Autodesk Inventor part; units mm, degrees
ref_plane "FDT_MOUNT_XY" through (0, 0, 8) normal (0, 0, 1) x (0, 1, 0)
ref_plane "FDT_MOUNT_YZ" through (0, 0, 8) normal (0, 1, 0) x (-1, 0, 0)
ref_plane "FDT_MOUNT_ZX" through (0, 0, 8) normal (-1, 0, 0) x (0, 0, 1)
sketch "Skizze_1" plane through (0, 0, 0) normal (0, 0, 1) x (1, 0, 0)
  line L0 (-14, 25) -> (-14, -25)
  line L1 (-14, -25) -> (14, -25)
  line L2 (14, -25) -> (14, 25)
  line L3 (14, 25) -> (-14, 25)
  circle A0 centre (0, 20) radius 2.75
  circle A1 centre (0, -20) radius 2.75
extrude "Extrusion1" add sketch "Skizze_1" along normal blind 8
sketch "Skizze_2_ALT_Drilling_1" plane through (0, 0, 0) normal (1, 0, 0) x (0, 1, 0)
  line L0 (0, 0) -> (0, 8)
  line L1 (0, 8) -> (7, 8)
  line L2 (7, 8) -> (6, 7)
  line L3 (6, 7) -> (6, 0)
  line L4 (6, 0) -> (0, 0)
  line L5 (0, 0) -> (0, 8)
revolve "Revolution1" cut sketch "Skizze_2_ALT_Drilling_1" angle 360 about axis through (0, 0, 0) along (0, 0, -1)
sketch "Skizze_3_ALT_Drilling_2" plane through (8, 0, 0) normal (1, 0, 0) x (0, 0, -1)
  line L0 (0, 8) -> (-8, 8)
  line L1 (-8, 8) -> (-8, 10.4)
  line L2 (-8, 10.4) -> (-5, 10.4)
  line L3 (-5, 10.4) -> (-5, 12)
  line L4 (-5, 12) -> (0, 12)
  line L5 (0, 12) -> (0, 8)
  line L6 (0, 8) -> (-8, 8)
revolve "Revolution2" cut sketch "Skizze_3_ALT_Drilling_2" angle 360 about axis through (8, 8, 0) along (0, 0, -1)
sketch "Muster_1_SKETCH_1" plane through (-8, 0, 0) normal (1, 0, 0) x (0, 0, -1)
  line L0 (0, 8) -> (-8, 8)
  line L1 (-8, 8) -> (-8, 10.4)
  line L2 (-8, 10.4) -> (-5, 10.4)
  line L3 (-5, 10.4) -> (-5, 12)
  line L4 (-5, 12) -> (0, 12)
  line L5 (0, 12) -> (0, 8)
  line L6 (0, 8) -> (-8, 8)
sketch "Muster_1_SKETCH_2" plane through (8, 0, 0) normal (1, 0, 0) x (0, 0, -1)
  line L0 (0, -8) -> (-8, -8)
  line L1 (-8, -8) -> (-8, -5.6)
  line L2 (-8, -5.6) -> (-5, -5.6)
  line L3 (-5, -5.6) -> (-5, -4)
  line L4 (-5, -4) -> (0, -4)
  line L5 (0, -4) -> (0, -8)
  line L6 (0, -8) -> (-8, -8)
sketch "Muster_1_SKETCH_3" plane through (-8, 0, 0) normal (1, 0, 0) x (0, 0, -1)
  line L0 (0, -8) -> (-8, -8)
  line L1 (-8, -8) -> (-8, -5.6)
  line L2 (-8, -5.6) -> (-5, -5.6)
  line L3 (-5, -5.6) -> (-5, -4)
  line L4 (-5, -4) -> (0, -4)
  line L5 (0, -4) -> (0, -8)
  line L6 (0, -8) -> (-8, -8)
revolve "Revolution3" cut sketch "Muster_1_SKETCH_1" angle 360 about axis through (-8, 8, 0) along (0, 0, -1)
revolve "Revolution4" cut sketch "Muster_1_SKETCH_2" angle 360 about axis through (8, -8, 0) along (0, 0, -1)
revolve "Revolution5" cut sketch "Muster_1_SKETCH_3" angle 360 about axis through (-8, -8, 0) along (0, 0, -1)
ref_plane "FDT_MOUNT_XY" through (0, 0, 8) normal (0, 0, 1) x (0, 1, 0)
ref_plane "FDT_MOUNT_YZ" through (0, 0, 8) normal (0, 1, 0) x (-1, 0, 0)
ref_plane "FDT_MOUNT_ZX" through (0, 0, 8) normal (-1, 0, 0) x (0, 0, 1)
ref_plane "FNC_1_XY" through (0, 0, 4) normal (0, 0, 1) x (1, 0, 0)
ref_plane "FNC_1_YZ" through (0, 0, 4) normal (1, 0, 0) x (0, 1, 0)
ref_plane "FNC_1_ZX" through (0, 0, 4) normal (0, 1, 0) x (0, 0, 1)
ref_plane "FNC_2_3_XY" through (0, 0, 8) normal (0, 0, 1) x (1, 0, 0)
ref_plane "FNC_2_3_YZ" through (0, 0, 8) normal (1, 0, 0) x (0, 1, 0)
ref_plane "FNC_2_3_ZX" through (0, 0, 8) normal (0, 1, 0) x (0, 0, 1)
ref_plane "FNC_Schraube_1_XY" through (-8, 8, 5) normal (0, 0, 1) x (1, 0, 0)
ref_plane "FNC_Schraube_1_YZ" through (-8, 8, 5) normal (1, 0, 0) x (0, 1, 0)
ref_plane "FNC_Schraube_1_ZX" through (-8, 8, 5) normal (0, 1, 0) x (0, 0, 1)
ref_plane "FNC_Schraube_2_XY" through (8, 8, 5) normal (0, 0, 1) x (1, 0, 0)
ref_plane "FNC_Schraube_2_YZ" through (8, 8, 5) normal (1, 0, 0) x (0, 1, 0)
ref_plane "FNC_Schraube_2_ZX" through (8, 8, 5) normal (0, 1, 0) x (0, 0, 1)
ref_plane "FNC_Schraube_3_XY" through (-8, -8, 5) normal (0, 0, 1) x (1, 0, 0)
ref_plane "FNC_Schraube_3_YZ" through (-8, -8, 5) normal (1, 0, 0) x (0, 1, 0)
ref_plane "FNC_Schraube_3_ZX" through (-8, -8, 5) normal (0, 1, 0) x (0, 0, 1)
ref_plane "FNC_Schraube_4_XY" through (8, -8, 5) normal (0, 0, 1) x (1, 0, 0)
ref_plane "FNC_Schraube_4_YZ" through (8, -8, 5) normal (1, 0, 0) x (0, 1, 0)
ref_plane "FNC_Schraube_4_ZX" through (8, -8, 5) normal (0, 1, 0) x (0, 0, 1)
ref_plane "P17_1_XY" through (0, 20, 8) normal (0, 0, 1) x (1, 0, 0)
ref_plane "P17_1_YZ" through (0, 20, 8) normal (1, 0, 0) x (0, 1, 0)
ref_plane "P17_1_ZX" through (0, 20, 8) normal (0, 1, 0) x (0, 0, 1)
ref_plane "P18_1_XY" through (0, -20, 8) normal (0, 0, 1) x (1, 0, 0)
ref_plane "P18_1_YZ" through (0, -20, 8) normal (1, 0, 0) x (0, 1, 0)
ref_plane "P18_1_ZX" through (0, -20, 8) normal (0, 1, 0) x (0, 0, 1)
properties part number "537245 FNC-12---(F)"
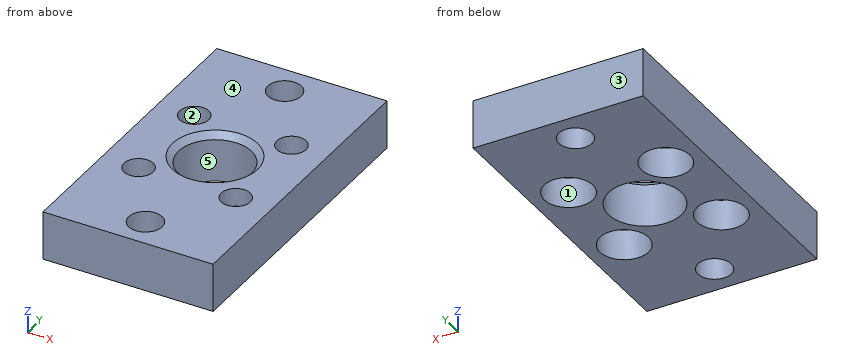
Check sheet for the modelled part. Datum: model origin and axes. Units: mm. Face numbers are marked on the shaded views. A direction names the side the tool comes from. Round coordinates to 2 decimals unless told otherwise and drop trailing zeros. Order: outer loops, then holes, each group sorted by start corner. A loop starts at its lowest first (then second) coordinate and runs counter-clockwise, first axis right, second up.
Q1. Depth check by flat-ended pin: P1, Ø5, axis at x = -8, y = -8, coming from the -Z side; P2, Ø4, axis at x = 6, y = 6.5, coming from the -Z side; P3, Ø4.5, axis at x = 0, y = 20, coming from the +Z side. Enter the tip coordinate at first touch or a pass-through.
Filled sheet:
P1: stops at z = 5
P2: stops at z = 0
P3: passes through
Q2. Cross-section at B-B, the plane z = 6. Enter the section's corners in (x, y), plus the area to 3 significant figures.
Filled sheet:
outline: (-14, -25) - (14, -25) - (14, 25) - (-14, 25) - close; hole circle Ø4.8 at (-8, -8); hole circle Ø4.8 at (-8, 8); hole circle Ø12 at (0, 0); hole circle Ø5.5 at (0, -20); hole circle Ø5.5 at (0, 20); hole circle Ø4.8 at (8, -8); hole circle Ø4.8 at (8, 8)
area: 1,170 mm2
Q3. Cross-section at C-C, the plane x = 0. Enter the section's corners in (y, z), plus the area to 3 significant figures.
Filled sheet:
outline: (-25, 0) - (-22.75, 0) - (-22.75, 8) - (-25, 8) - close; (-17.25, 0) - (-6, 0) - (-6, 7) - (-7, 8) - (-17.25, 8) - close; (6, 0) - (17.25, 0) - (17.25, 8) - (7, 8) - (6, 7) - close; (22.75, 0) - (25, 0) - (25, 8) - (22.75, 8) - close
area: 215 mm2
Q4. Cross-section at A-A, the plane y = -8. Enter the section's corners in (x, z).
Filled sheet:
outline: (-14, 0) - (-12, 0) - (-12, 5) - (-10.4, 5) - (-10.4, 8) - (-14, 8) - close; (-5.6, 5) - (-4, 5) - (-4, 0) - (4, 0) - (4, 5) - (5.6, 5) - (5.6, 8) - (-5.6, 8) - close; (10.4, 5) - (12, 5) - (12, 0) - (14, 0) - (14, 8) - (10.4, 8) - close
Q5. Cross-section at D-D, the plane y = -20. Enter the section's corners in (x, z), plus the area to 3 significant figures.
Filled sheet:
outline: (-14, 0) - (-2.75, 0) - (-2.75, 8) - (-14, 8) - close; (2.75, 0) - (14, 0) - (14, 8) - (2.75, 8) - close
area: 180 mm2
Q6. Set-up check for the marked faces 1 and 2: record each of +Z, -Z, +X, -X, +Y, -Y from which the full face is reachable in a straight line by a thin tool's end or side.
Filled sheet:
face 1: -Z
face 2: +Z, -Z
Q7. Draft check along Y on the marked faces 3, 4 and 5. Enter one of: pulls with the +Y half, pulls with the -Y half, needs draft (parallel to the pull), parting line crosses it, or undercut.
Filled sheet:
face 3: pulls with the +Y half
face 4: needs draft
face 5: undercut
Q8. Scan lines: L1, parallel to X at y = -8, z = 6.8; L2, parallel to X at y = 8, z = 3.7; L3, parallel to Y at x = 0.75, z = 6.5. Record each from-to range of solid material in increasing order.
Filled sheet:
L1: x = -14 to -10.4, -5.6 to 5.6, 10.4 to 14
L2: x = -14 to -12, -4 to 4, 12 to 14
L3: y = -25 to -22.65, -17.35 to -5.95, 5.95 to 17.35, 22.65 to 25
